Part model, mm, in its own coordinate system. Coordinates: 2 decimals unless noted, no trailing zeros. Write each loop counter-clockwise with the first axis right and the second up, starting at its lowest first coordinate (ties: lowest second). Pieces come first, ordered by that corner, then holes. Notation, with made-up numbers: (81.5, 82.25) -> (118.5, 82.25) arc R19 ccw to (118.5, 100.25) -> close; hole circle Ø9 at (67.25, 88). An arc over 180 degrees is marked (long way). Write item = value, one per line. Start each with the question number.
Q1. Band-saw the part on B-B, the plane z = 2.5. Give the number of separate pieces and of enclosed holes in the cut face, plus the area to 3 significant figures.
Q2. Probe line 1 (Y direction, x = 0, z = 4.65) (3 decimals); line 2 (Y direction, x = 47, z = 2.5); line 3 (X direction, y = -27, z = 1.5). List the from-to ranges inside material, lowest first.
Q3. Band-saw the part on A-A, the plane x = 0. List the corners of the cut face in (y, z) (3 decimals), plus the area to 3 significant figures.
Q4. Pin check, flat tips, straight feed: P1, Ø2, axis at x = 21.5, z = 2, coming from the -Y side; P2, Ø2, axis at x = 47.5, z = 5, coming from the -Y side; P3, Ø3, axis at y = 5, z = 1.5, coming from the +X side. Stop position of each tip, or through.
Q5. Pull direction X, two halves, no side cores. Call faces 1 (the cylindrical face through (-60.15, 0.18, 3.29)), 2 (the cylindrical face through (-45.22, 27.47, 3.04)), 3 (the cylindrical face through (-0.98, -57.14, 3.21)): released by +X, released by -X, zero draft, split by the parting line, or undercut.
from build123d import *

# Parameters (mm, degrees)
EXTRUDE_1_DEPTH             = 6
CUT_EXTRUDE_1_DEPTH         = 7
HOLE_WIZARD_3_2_3_2_1_D     = 3.2
HOLE_WIZARD_3_2_3_2_1_DEPTH = 6
FILLET_1_R                  = 5
CHAMFER_1_SIZE              = 0.5


with BuildPart() as part:
    # 草图1 → 凸台-拉伸1 (new body)
    with BuildSketch(Plane.XY.offset(6)):
        with BuildLine():
            Line((-54.404710274, 17.5), (-58.249656651, 15))
            ThreePointArc((-58.249656651, 15), (0, -60.15), (58.249656651, 15))
            Line((58.249656651, 15), (54.404710274, 17.5))
            ThreePointArc((54.404710274, 17.5), (0, 57.15), (-54.404710274, 17.5))
        make_face()
    extrude(amount=-EXTRUDE_1_DEPTH)

    # 草图2 → 切除-拉伸1 (cut, through all)
    with BuildSketch(Plane(origin=(0, 0, 0), x_dir=(-1, 0, 0), z_dir=(0, 0, -1))):
        with BuildLine():
            Line((58.249656651, -15), (54.404710274, -17.5))
            ThreePointArc((54.404710274, -17.5), (0, -57.15), (-54.404710274, -17.5))
            Line((-54.404710274, -17.5), (-58.249656651, -15))
            ThreePointArc((-58.249656651, -15), (0, -60.15), (58.249656651, -15))
        make_face()
    extrude(amount=-CUT_EXTRUDE_1_DEPTH, mode=Mode.SUBTRACT)

    # Ø3.2 (3.2) 直径孔1
    with Locations(Plane(origin=(0, 0, 0), x_dir=(-1, 0, 0), z_dir=(0, 0, -1))):
        with Locations((0, 53.975), (46.743721169, -26.9875), (-46.743721169, 26.9875), (-46.743721169, -26.9875), (0, -53.975), (46.743721169, 26.9875)):
            Hole(HOLE_WIZARD_3_2_3_2_1_D / 2, depth=HOLE_WIZARD_3_2_3_2_1_DEPTH)

    # 圆角1
    fillet_1_edges = [part.edges().sort_by_distance(p)[0] for p in [
        (-58.249656651, -15, 3),
        (58.249656651, -15, 3),
        (54.404710274, -17.5, 3),
        (-54.404710274, -17.5, 3),
        (54.404710274, 17.5, 3),
        (58.249656651, 15, 3),
        (-58.249656651, 15, 3),
        (-54.404710274, 17.5, 3),
    ]]
    fillet(fillet_1_edges, radius=FILLET_1_R)

    # 倒角1
    chamfer_1_edges = [part.edges().sort_by_distance(p)[0] for p in [
        (0, -57.15, 0),
        (-56.218559502, -16.320627747, 0),
        (60.15, 0, 0),
        (56.218559502, 16.320627747, 0),
        (56.218559502, -16.320627747, 0),
        (-60.15, 0, 0),
        (-56.218559502, 16.320627747, 0),
        (0, 57.15, 0),
        (-57.961950962, 14.742761538, 0),
        (57.961950962, -14.742761538, 0),
        (-57.961950962, -14.742761538, 0),
        (57.961950962, 14.742761538, 0),
        (-54.657828511, -17.651398409, 0),
        (54.657828511, -17.651398409, 0),
        (54.657828511, 17.651398409, 0),
        (-54.657828511, 17.651398409, 0),
    ]]
    chamfer(chamfer_1_edges, length=CHAMFER_1_SIZE)


solid = part.part
Ans:
q1.separate_pieces = 1
q1.enclosed_holes = 6
q1.area = 10,400 mm2
q2.line_1 = -57.15 to -55.575, -52.375 to 52.375, 55.575 to 57.15
q2.line_2 = -32.51 to -28.57, -25.41 to 25.41, 28.57 to 32.51
q2.line_3 = -50.37 to -48.34, -45.14 to 45.14, 48.34 to 50.37
q3.outline = (-57.15, 0.5) -> (-56.65, 0) -> (-55.575, 0) -> (-55.575, 6) -> (-57.15, 6) -> close; (-52.375, 0) -> (52.375, 0) -> (52.375, 6) -> (-52.375, 6) -> close; (55.575, 0) -> (56.65, 0) -> (57.15, 0.5) -> (57.15, 6) -> (55.575, 6) -> close
q3.area = 647 mm2
q4.P1 = -53.35
q4.P2 = -33.22
q4.P3 = 60.05
q5.face_1 = released by -X
q5.face_2 = undercut
q5.face_3 = split by the parting line
